Here's the drawing with two shaded views (mm, measured from the low corner). I have some questions. A direction names the side the tool comes from. Give positions to 0.01 mm unless a question says otherwise; leave off trailing zeros. Write each loop counter-clockwise with the first axis right and the second up, starting at its lowest first coordinate (ties: lowest second). Pieces come first, ordered by that corner, then holes.
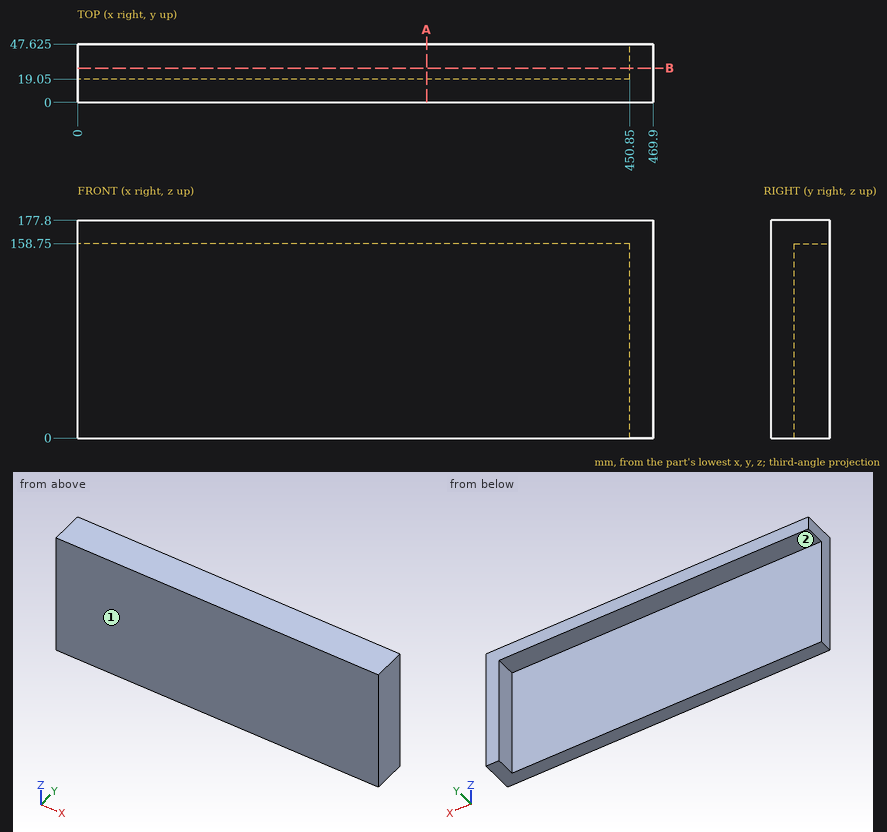
(1) Imagine slicing it at A-A, the plane x = 285. Write out the boundary of the cut face in (y, z) (3 decimals).
Returned:
outline: (0, 0) - (19.05, 0) - (19.05, 158.75) - (47.625, 158.75) - (47.625, 177.8) - (0, 177.8) - close
(2) For the marked faces 1 and 2, which set-ups out of +Z, -Z, +X, -X, +Y, -Y let a thin tool reach every point of the face, with its end or its side?
Returned:
face 1: +Z, -Z, +X, -X, -Y
face 2: -Z, -X, +Y
(3) Will these pins go through, and if not, where does the flat tip stop? P1, Ø12, axis at x = 226, y = 29.5, coming from the -Z side; P2, Ø14.5, axis at y = 29.5, z = 102.5, coming from the -X side; P3, Ø5, axis at x = 102, z = 127.5, coming from the +Y side; P4, Ø23, axis at x = 199.5, y = 27.5, coming from the -Z side.
Returned:
P1: stops at z = 158.75
P2: stops at x = 450.85
P3: stops at y = 19.05
P4: stops at z = 0
(4) If I drill on L1, parallel to X at y = 22, z = 136; L2, parallel to Z at x = 212.5, y = 27; L3, parallel to Y at x = 136.5, z = 117, over which ranges is the centre line in solid material (lowest first)?
Returned:
L1: x = 450.85 to 469.9
L2: z = 158.75 to 177.8
L3: y = 0 to 19.05
(5) Imagine slicing it at B-B, the plane y = 28. Write out the boundary of the cut face in (x, z), plus the area to 3 significant figures.
Returned:
outline: (0, 158.75) - (450.85, 158.75) - (450.85, 0) - (469.9, 0) - (469.9, 177.8) - (0, 177.8) - close
area: 12,000 mm2
